Geometry: final body of the model. Coordinates: model frame, mm. A direction names the side the tool comes from. Coordinates: 2 decimals unless noted, no trailing zeros. Write each loop counter-clockwise with the first axis right and the second up, starting at its lowest first coordinate (ties: lowest second). Pieces come first, ordered by that corner, then holes. Notation, with made-up numbers: (25.5, 49.25) - (46.5, 49.25) arc R12 cw to (46.5, 63.25) - close; hole circle Ø6 at (-34, 26.25). An arc over 180 degrees is marked (long way). Put each result on its own line as item: value.
```python
from build123d import *

# Parameters (mm, degrees)
BOSS_EXTRUDE1_DEPTH                  = 15
BOSS_EXTRUDE2_START                  = 6
SKETCH1_3_R                          = 6
BOSS_EXTRUDE2_DEPTH                  = 9
BOSS_EXTRUDE3_START                  = -15
SKETCH1_4_R                          = 6
BOSS_EXTRUDE3_DEPTH                  = 9
FILLET1_RADIUS                       = 15
FILLET1_LENGTH                       = 9
FILLET2_RADIUS                       = 15
FILLET2_LENGTH                       = 9
F_12_0MM_DOWEL_HOLE1_D               = 12
F_12_0MM_DOWEL_HOLE1_DEPTH           = 13
F_12_0MM_DOWEL_HOLE1_ON_FACE_2_D     = 12
F_12_0MM_DOWEL_HOLE1_ON_FACE_2_DEPTH = 13
FILLET6_R                            = 1
FILLET4_R                            = 1
FILLET5_R                            = 1
FILLET7_R                            = 1


with BuildPart() as part:
    # Sketch1 → Boss-Extrude1 (new, symmetric)
    with BuildSketch(Plane.XY):
        Polygon((0, 45), (0, 0), (9, 0), (9, 36), (60, 36), (60, 45), (30, 45), align=None)
    extrude(amount=BOSS_EXTRUDE1_DEPTH, both=True)

    # Sketch1<3> → Boss-Extrude2 (add)
    with BuildSketch(Plane.XY.offset(BOSS_EXTRUDE2_START)):
        with BuildLine():
            Line((0, 60), (0, 45))
            Line((0, 45), (30, 45))
            Line((30, 45), (30, 60))
            ThreePointArc((30, 60), (15, 75), (0, 60))
        make_face()
        with Locations((15, 60)):
            Circle(SKETCH1_3_R, mode=Mode.SUBTRACT)
    extrude(amount=BOSS_EXTRUDE2_DEPTH)

    # Sketch1<4> → Boss-Extrude3 (add)
    with BuildSketch(Plane.XY.offset(BOSS_EXTRUDE3_START)):
        with BuildLine():
            Line((0, 60), (0, 45))
            Line((0, 45), (30, 45))
            Line((30, 45), (30, 60))
            ThreePointArc((30, 60), (15, 75), (0, 60))
        make_face()
        with Locations((15, 60)):
            Circle(SKETCH1_4_R, mode=Mode.SUBTRACT)
    extrude(amount=BOSS_EXTRUDE3_DEPTH)

    # Fillet1: full round fillet: the end face becomes a half cylinder, R = half its width
    fillet1_face = Plane((60, 40.5, 0), x_dir=(0, -1, 0), z_dir=(1, 0, 0))  # on the end face: x along it, z out of the body
    fillet1_slab = fillet1_face.offset(-FILLET1_RADIUS / 2) * Box(FILLET1_LENGTH, 2 * FILLET1_RADIUS, FILLET1_RADIUS, mode=Mode.PRIVATE)  # the body's end, R deep
    fillet1_round = Plane((45, 40.5, 0), x_dir=(1, 0, 0), z_dir=(0, -1, 0)) * Cylinder(FILLET1_RADIUS, FILLET1_LENGTH, mode=Mode.PRIVATE)  # its axis R under the face
    add(fillet1_slab - fillet1_round, mode=Mode.SUBTRACT)

    # Fillet2: full round fillet: the end face becomes a half cylinder, R = half its width
    fillet2_face = Plane((4.5, 0, 0), x_dir=(1, 0, 0), z_dir=(0, -1, 0))  # on the end face: x along it, z out of the body
    fillet2_slab = fillet2_face.offset(-FILLET2_RADIUS / 2) * Box(FILLET2_LENGTH, 2 * FILLET2_RADIUS, FILLET2_RADIUS, mode=Mode.PRIVATE)  # the body's end, R deep
    fillet2_round = Plane((4.5, 15, 0), x_dir=(0, -1, 0), z_dir=(1, 0, 0)) * Cylinder(FILLET2_RADIUS, FILLET2_LENGTH, mode=Mode.PRIVATE)  # its axis R under the face
    add(fillet2_slab - fillet2_round, mode=Mode.SUBTRACT)

    # Ø12.0mm Dowel Hole1
    with Locations(Plane(origin=(45, 45, 0), x_dir=(1, 0, 0), z_dir=(0, 1, 0))):
        with Locations((0, 0)):
            Hole(F_12_0MM_DOWEL_HOLE1_D / 2, depth=F_12_0MM_DOWEL_HOLE1_DEPTH)

    # Ø12.0mm Dowel Hole1 on face 2
    with Locations(Plane(origin=(9, 15, 0), x_dir=(0, 0, 1), z_dir=(1, 0, 0))):
        with Locations((0, 0)):
            Hole(F_12_0MM_DOWEL_HOLE1_ON_FACE_2_D / 2, depth=F_12_0MM_DOWEL_HOLE1_ON_FACE_2_DEPTH)

    # Fillet6
    fillet6_edges = [part.edges().sort_by_distance(p)[0] for p in [
        (9, 36, 0),
    ]]
    fillet(fillet6_edges, radius=FILLET6_R)

    # Fillet4
    fillet4_edges = [part.edges().sort_by_distance(p)[0] for p in [
        (30, 45, -10.5),
    ]]
    fillet(fillet4_edges, radius=FILLET4_R)

    # Fillet5
    fillet5_edges = [part.edges().sort_by_distance(p)[0] for p in [
        (30, 45, 10.5),
    ]]
    fillet(fillet5_edges, radius=FILLET5_R)

    # Fillet7
    fillet7_edges = [part.edges().sort_by_distance(p)[0] for p in [
        (15.5, 45, -6),
        (15.5, 45, 6),
    ]]
    fillet(fillet7_edges, radius=FILLET7_R)


solid = part.part
```
1. Section query A-A (z = 0). Return loops of the section in (x, y), then the cut area to 3 significant figures.
Answer below:
outline: (0, 0) - (9, 0) - (9, 9) - (0, 9) - close; (0, 21) - (9, 21) - (9, 35) arc R1 cw to (10, 36) - (39, 36) - (39, 45) - (0, 45) - close; (51, 36) - (60, 36) - (60, 45) - (51, 45) - close
area: 648 mm²
2. Mould query, pull axis Z, two halves, no side actions, for faces 4 (the flat face through (17, 45, 15)), 5 (the cylindrical face through (51, 40, 0)), 6 (the flat face through (30, 53, -11)). Classes: +Z half, -Z half, draft (parallel to the pull), parting line (faces both ways), or undercut.
Answer below:
face 4: +Z half
face 5: undercut
face 6: draft
3. Pin query (flat end, axial travel): pin 1 Ø9.5 at (x, z) = (45, 0) entering from -Y; pin 2 Ø1 at (x, z) = (22.5, -7.5) entering from -Y; pin 3 Ø14 at (x, y) = (15, 60) entering from -Z; pin 4 Ø7 at (y, z) = (50.5, 11) entering from +X. Return the tip coordinate at first contact, or that it passes through.
Answer below:
pin 1: passes through
pin 2: stops at y = 36
pin 3: stops at z = -15
pin 4: stops at x = 30
4. Set-up query: faces 1 (the flat face through (9, 21, 4)), 2 (the flat face through (18, 54, -6)), 3 (the flat face through (37, 45, 0)). Return all of +Z, -Z, +X, -X, +Y, -Y with unobstructed straight access to the full face (end or side cutting, diameter ignored); none if empty.
Answer below:
face 1: +Z, -Z, +X, -Y
face 2: +X, -X, +Y
face 3: +X, +Y
5. Ray query, probe 1 along Y at (x, z) = (15, 10); probe 2 along Y at (x, z) = (2.25, 0); probe 3 along Z at (x, y) = (45, 38.75). Return the intervals inside material, ascending. Write a range as from..to.
Answer below:
probe 1: y = 36..54, 66..75
probe 2: y = 0..9, 21..45
probe 3: z = -15..-6, 6..15
6. Section query B-B (y = 13). Return loops of the section in (x, z), then the cut area to 3 significant figures.
Answer below:
outline: (0, -14.87) - (9, -14.87) - (9, -5.66) - (0, -5.66) - close; (0, 5.66) - (9, 5.66) - (9, 14.87) - (0, 14.87) - close
area: 166 mm²
7. Section query C-C (x = 7.5). Return loops of the section in (y, z), then the cut area to 3 significant figures.
Answer below:
outline: (15, -15) - (72.99, -15) - (72.99, -6) - (46, -6) arc R1 cw to (45, -5) - (45, 5) arc R1 cw to (46, 6) - (72.99, 6) - (72.99, 15) - (15, 15) arc R15 ccw to start; hole circle Ø12 at (15, 0)
area: 1,640 mm²
8. Section query D-D (z = -12). Return loops of the section in (x, y), then the cut area to 3 significant figures.
Answer below:
outline: (0, 6) - (9, 6) - (9, 35) arc R1 cw to (10, 36) - (54, 36) - (54, 45) - (31, 45) arc R1 cw to (30, 46) - (30, 60) arc R15 ccw to (0, 60) - close; hole circle Ø12 at (15, 60)
area: 1,450 mm²
